from build123d import *

# Parameters (mm, degrees)
F1_DEPTH = 5.842


with BuildPart() as f1:
    # F0 (on Front) → F1 (new body)
    with BuildSketch(Plane.XZ):
        Polygon((0, 6.35), (0, 0), (12.7, 0), (22.86, 0), (33.02, 0), (43.18, 0), (53.34, 0), (63.5, 0), (63.5, 6.35), align=None)
        Polygon((22.86, 0), (12.7, 0), (12.7, -4.7625), align=None)
        Polygon((33.02, 0), (22.86, 0), (22.86, -4.7625), align=None)
        Polygon((43.18, 0), (33.02, 0), (33.02, -4.7625), align=None)
        Polygon((53.34, -4.7625), (63.5, 0), (53.34, 0), align=None)
        Polygon((53.34, 0), (43.18, 0), (43.18, -4.7625), align=None)
    extrude(amount=F1_DEPTH)


solid = f1.part
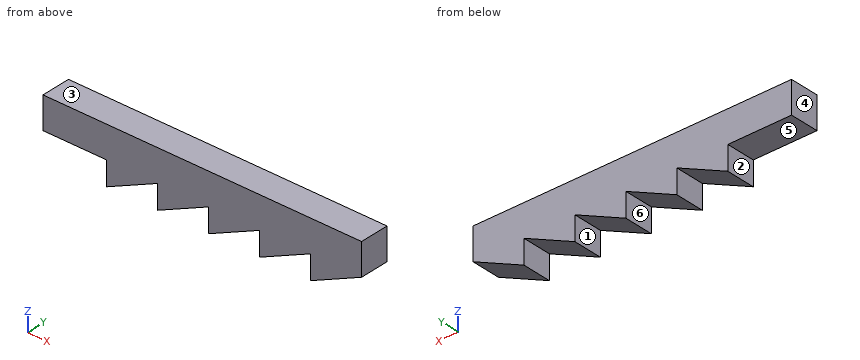
Could you check a few things on this model? Use its own coordinates, in mm. Face numbers are marked on the shaded views. A direction names the side the tool comes from. Coordinates: 2 decimals unless noted, no trailing zeros. Write each loop counter-clockwise with the first axis right and the second up, starting at its lowest first coordinate (ties: lowest second). Pieces come first, ordered by that corner, then holes. Notation, with made-up numbers: M 41,-21 L 73,-21 A24 ccw 73,4 Z; hole C -24,45.5 d5. An arc over 180 degrees is marked long. One line per question, with ' | ' between items.
1) If we mould it in two halves opening along X, with no side actions, what happens to the marked faces 1, 2 and 3? For each: released by +X, released by -X, zero draft, split by the parting line, or undercut.
Checks:
face 1: undercut | face 2: released by -X | face 3: zero draft
2) I need wall thicknesses on probe 1 along X at (y, z) = (-2.5, -1); probe 2 along Z at (x, y) = (8, -2); probe 3 along Z at (x, y) = (49.5, -2.85). Which ranges of each line are inside material? Lowest first, please. Write a range as [from, to].
Checks:
probe 1: [12.7, 20.73], [22.86, 30.89], [33.02, 41.05], [43.18, 51.21], [53.34, 61.37] | probe 2: [0, 6.35] | probe 3: [-1.8, 6.35]
3) Imagine slicing it at B-B, the plane y = -2.6. Write out the boundary of the cut face in (x, z), and give its area (3 significant figures).
Checks:
outline: M 0,0 L 12.7,0 L 12.7,-4.76 L 22.86,0 L 22.86,-4.76 L 33.02,0 L 33.02,-4.76 L 43.18,0 L 43.18,-4.76 L 53.34,0 L 53.34,-4.76 L 63.5,0 L 63.5,6.35 L 0,6.35 Z | area: 524 mm²
4) Imagine slicing it at C-C, the plane x = 12. Write out the boundary of the cut face in (y, z), and give its area (3 significant figures).
Checks:
outline: M -5.84,0 L 0,0 L 0,6.35 L -5.84,6.35 Z | area: 37.1 mm²
5) Imagine slicing it at D-D, the plane x = 28.5. Write out the boundary of the cut face in (y, z), and give its area (3 significant figures).
Checks:
outline: M -5.84,-2.12 L 0,-2.12 L 0,6.35 L -5.84,6.35 Z | area: 49.5 mm²
6) For the marked faces 4, 5 and 6, which set-ups out of +Z, -Z, +X, -X, +Y, -Y let a thin tool reach every point of the face, with its end or its side?
Checks:
face 4: +Z, -Z, -X, +Y, -Y | face 5: -Z, -X, +Y, -Y | face 6: -Z, +Y, -Y
7) For pin 1 Ø3 at (x, z) = (35, -2.5) entering from +Y; pin 2 Ø1.8 at (x, y) = (6, -3.5) entering from -Z; pin 3 Ø2.5 at (y, z) = (-2, -2.5) entering from -X, each with a flat end and sliding along its axis, tell me the tip position at first contact or that it passes through.
Checks:
pin 1: y = 0 | pin 2: z = 0 | pin 3: x = 12.7
8) Imagine slicing it at A-A, the plane z = -3. Write out the boundary of the cut face in (x, y).
Checks:
outline: M 12.7,-5.84 L 16.46,-5.84 L 16.46,0 L 12.7,0 Z; M 22.86,-5.84 L 26.62,-5.84 L 26.62,0 L 22.86,0 Z; M 33.02,-5.84 L 36.78,-5.84 L 36.78,0 L 33.02,0 Z; M 43.18,-5.84 L 46.94,-5.84 L 46.94,0 L 43.18,0 Z; M 53.34,-5.84 L 57.1,-5.84 L 57.1,0 L 53.34,0 Z
